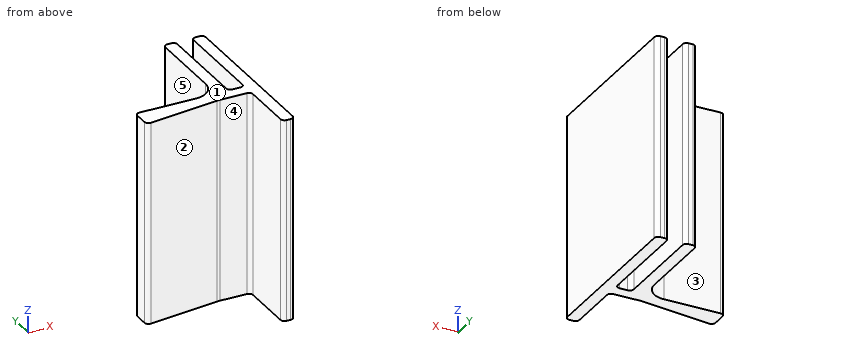
from build123d import *

# Parameters (mm, degrees)
F1_DEPTH = 50
F2_R     = 5
F3_R     = 1


with BuildPart() as f1:
    # F0 (on Top) → F1 (new body)
    with BuildSketch(Plane.XY):
        Polygon((0, 15), (0, 0), (3, 0), (3, 43), (0, 43), (0, 18), (-4, 18), (-4, 43), (-7, 43), (-7, 18), (-27, 18), (-27, 15), (-8, 15), align=None)
        Polygon((-27, 12.5), (-8, 15), (-27, 15), align=None)
    extrude(amount=F1_DEPTH)

    # F2
    f2_edges = [f1.edges().sort_by_distance(p)[0] for p in [
        (-8, 15, 25),
        (-7, 18, 25),
    ]]
    fillet(f2_edges, radius=F2_R)

    # F3
    f3_edges = [f1.edges().sort_by_distance(p)[0] for p in [
        (-7, 43, 25),
        (-4, 43, 25),
        (0, 43, 25),
        (3, 43, 25),
        (0, 0, 25),
        (3, 0, 25),
        (0, 15, 25),
        (-4, 18, 25),
        (0, 18, 25),
        (-27, 12.5, 25),
        (-27, 18, 25),
    ]]
    fillet(f3_edges, radius=F3_R)


solid = f1.part
Design review of the part built by this model. Coordinates are the model's own, in mm. Face numbers are marked on the shaded views. A direction names the side the tool comes from. Coordinates: 2 decimals unless noted, no trailing zeros. Order: outer loops, then holes, each group sorted by start corner. A loop starts at its lowest first (then second) coordinate and runs counter-clockwise, first axis right, second up. Notation, with made-up numbers: (31, -21) -> (37, -21) arc R15 cw to (37, -13) -> close; hole circle Ø8 at (29, 23). An arc over 180 degrees is marked (long way). One line per item, written item: value.
1) Machinability: for the marked faces 1 and 2, which of the approach directions +Z, -Z, +X, -X, +Y, -Y give a long, thin tool a straight path to every point of the face, cutting with its end or side? Answer none if there is none.
Output values:
face 1: +Z, +X, -X, +Y, -Y
face 2: +Z, -Z, -Y
2) Draft analysis for pull direction X (two halves, no side actions). For the marked faces 3, 4 and 5, state which applies: +X half, -X half, draft (parallel to the pull), parting line (faces both ways), or undercut.
Output values:
face 3: draft
face 4: undercut
face 5: -X half
3) We need section D-D, the plane x = -23.5. Give the boundary of the cut face in (y, z).
Output values:
outline: (12.96, 0) -> (18, 0) -> (18, 50) -> (12.96, 50) -> close
4) Clearance check with flat-ended pins moving along their axes: P1, Ø15, axis at y = 31, z = 18, coming from the -X side; P2, Ø1.5, axis at x = -12.5, z = 18.5, coming from the +Y side; P3, Ø6, axis at x = -6.5, y = 34, coming from the -Z side; P4, Ø11.5, axis at y = 27.5, z = 21, coming from the -X side. State where each tip first meets the part, or that it passes through.
Output values:
P1: stops at x = -7
P2: stops at y = 18.01
P3: stops at z = 0
P4: stops at x = -7.16
5) To check wall thickness, follow probe 1 along X at (y, z) = (35.5, 32.5); probe 2 along X at (y, z) = (3, 47.5); probe 3 along Y at (x, z) = (-1.5, 20). State the ranges of each line that lie inside material, in increasing order. Write a range as [from, to].
Output values:
probe 1: x = [-7, -4], [0, 3]
probe 2: x = [0, 3]
probe 3: y = [15, 18]
6) We need section C-C, the plane y = 8. Give the boundary of the cut face in (x, z), then the cut area to 3 significant figures.
Output values:
outline: (0, 0) -> (3, 0) -> (3, 50) -> (0, 50) -> close
area: 150 mm2
7) We need section A-A, the plane y = 28. Give the boundary of the cut face in (x, z), then the cut area to 3 significant figures.
Output values:
outline: (-7, 0) -> (-4, 0) -> (-4, 50) -> (-7, 50) -> close; (0, 0) -> (3, 0) -> (3, 50) -> (0, 50) -> close
area: 300 mm2
8) We need section B-B, the plane z = 7. Give the boundary of the cut face in (x, y), then the cut area to 3 significant figures.
Output values:
outline: (-27, 13.64) arc R1 ccw to (-25.87, 12.65) -> (-8.32, 14.96) arc R5 cw to (-7.67, 15) -> (-1, 15) arc R1 cw to (0, 14) -> (0, 1) arc R1 ccw to (1, 0) -> (2, 0) arc R1 ccw to (3, 1) -> (3, 42) arc R1 ccw to (2, 43) -> (1, 43) arc R1 ccw to (0, 42) -> (0, 19) arc R1 cw to (-1, 18) -> (-3, 18) arc R1 cw to (-4, 19) -> (-4, 42) arc R1 ccw to (-5, 43) -> (-6, 43) arc R1 ccw to (-7, 42) -> (-7, 23) arc R5 cw to (-12, 18) -> (-26, 18) arc R1 ccw to (-27, 17) -> close
area: 313 mm2
